Autodesk Inventor part; units mm, degrees
ref_plane "YZ Plane" through (0, 0, 0) normal (1, 0, 0) x (0, 1, 0)
ref_plane "XZ Plane" through (0, 0, 0) normal (0, 1, 0) x (-1, 0, 0)
ref_plane "XY Plane" through (0, 0, 0) normal (0, 0, 1) x (1, 0, 0)
sketch "Skizze1" plane through (0, 0, 0) normal (0, 0, 1) x (1, 0, 0)
  line L0 (0, 0) -> (242, 0)
  line L1 (242, 0) -> (242, 85)
  line L2 (242, 85) -> (0, 85)
  line L3 (0, 85) -> (0, 0)
  line L4 (242, 42.5) -> (842, 42.5)
  line L5 (0, 42.5) -> (-937, 42.5)
  arc A0 (240, 0) -> (240, 85) centre (-210.5625, 42.5) ccw
  arc A1 (2, 85) -> (2, 0) centre (452.5625, 42.5) ccw
  dimension "d0" = 85
  dimension "d1" = 242
  dimension "d2" = 2
  dimension "d3" = 2
  dimension "d4" = 2
  dimension "d7" = 452.5625
  dimension "d8" = 452.5625
extrude "Extrusion1" add sketch "Skizze1" against normal blind 2.5 contours A1 L2 A0 L0
sketch "Skizze2" plane through (0, 0, 0) normal (0, 0, 1) x (1, 0, 0)
  line L0 (2, 0) -> (240, 0)
  line L1 (240, 85) -> (2, 85)
  line L2 (121, 0) -> (121, 85)
  point P0 (0, 0)
  point P1 (3.1, 42.5)
  point P2 (238.9, 42.5)
  dimension "d11" = 42.5
  dimension "d12" = 42.5
  dimension "d13" = 235.8
  dimension "d14" = 117.9
  dimension "d15" = 117.9
hole "Bohrung1" at (3.1, 42.5, 0) at (238.9, 42.5, 0) direction (0, 0, -1) diameter 3.3 depth 8 tip angle 118
sketch "Skizze3" plane through (0, 0, 0) normal (0, 0, 1) x (1, 0, 0)
  line L0 (2, 0) -> (240, 0)
  line L1 (240, 85) -> (2, 85)
  arc A0 (2, 85) -> (2, 0) centre (452.5625, 42.5) ccw
  line L2 (8.1386, 91.5936) -> (-1.2688, 78.1585)
  line L3 (-1.2688, 78.1585) -> (-1.2688, 91.5936)
  line L4 (-1.2688, 91.5936) -> (8.1386, 91.5936)
  line L5 (-1.7926, 7.5896) -> (9.0296, -7.8661)
  line L6 (9.0296, -7.8661) -> (-1.7926, -7.8661)
  line L7 (-1.7926, -7.8661) -> (-1.7926, 7.5896)
  line L8 (121, 0) -> (121, 85)
  line L9 (233.8614, 91.5936) -> (243.2688, 78.1585)
  line L10 (243.2688, 78.1585) -> (243.2688, 91.5936)
  line L11 (243.2688, 91.5936) -> (233.8614, 91.5936)
  line L12 (243.7926, 7.5896) -> (232.9704, -7.8661)
  line L13 (232.9704, -7.8661) -> (243.7926, -7.8661)
  line L14 (243.7926, -7.8661) -> (243.7926, 7.5896)
  point P0 (0, 0)
  point P1 (1.7712, 82.5)
  point P2 (1.7712, 2.5)
  point P3 (242, 0)
  point P4 (240.2288, 82.5)
  point P5 (240.2288, 2.5)
  dimension "d23" = 55
  dimension "d24" = 55
  dimension "d25" = 2.5
  dimension "d26" = 2.5
extrude "Extrusion2" cut sketch "Skizze3" against normal blind 5 contours A0 L5 L0 | L0 L5 L6 L7 A0 | L9 L11 L10 | L12 L14 L13 | L2 L3 L4 L1 A0 | A0 L1 L2
sketch "Sketch7" plane through (0, 0, 0) normal (0, 0, 1) x (1, 0, 0)
  point P0 (0, 0)
sketch "Sketch9" plane through (0, 0, -2.5) normal (0, 0, -1) x (-1, 0, 0)
  line L0 (-238.4783, 85) -> (-3.5217, 85)
  line L1 (-214.9283, 63.0506) -> (-222.0283, 63.0506) construction
  line L2 (-222.0283, 63.0506) -> (-222.0283, 66.9494)
  line L3 (-222.0283, 66.9494) -> (-214.9283, 66.9494) construction
  line L4 (-214.9283, 66.9494) -> (-214.9283, 63.0506)
  line L5 (-214.9283, 63.0506) -> (-222.0283, 66.9494) construction
  line L6 (-222.0283, 63.0506) -> (-214.9283, 66.9494) construction
  arc A0 (-222.0283, 63.0506) -> (-214.9283, 63.0506) centre (-218.4783, 65) ccw
  arc A1 (-214.9283, 66.9494) -> (-222.0283, 66.9494) centre (-218.4783, 65) ccw
  line L7 (-194.9283, 63.0506) -> (-202.0283, 63.0506) construction
  line L8 (-202.0283, 63.0506) -> (-202.0283, 66.9494)
  line L9 (-202.0283, 66.9494) -> (-194.9283, 66.9494) construction
  line L10 (-194.9283, 66.9494) -> (-194.9283, 63.0506)
  line L11 (-194.9283, 63.0506) -> (-202.0283, 66.9494) construction
  line L12 (-202.0283, 63.0506) -> (-194.9283, 66.9494) construction
  arc A2 (-202.0283, 63.0506) -> (-194.9283, 63.0506) centre (-198.4783, 65) ccw
  arc A3 (-194.9283, 66.9494) -> (-202.0283, 66.9494) centre (-198.4783, 65) ccw
  line L13 (-174.9283, 63.0506) -> (-182.0283, 63.0506) construction
  line L14 (-182.0283, 63.0506) -> (-182.0283, 66.9494)
  line L15 (-182.0283, 66.9494) -> (-174.9283, 66.9494) construction
  line L16 (-174.9283, 66.9494) -> (-174.9283, 63.0506)
  line L17 (-174.9283, 63.0506) -> (-182.0283, 66.9494) construction
  line L18 (-182.0283, 63.0506) -> (-174.9283, 66.9494) construction
  arc A4 (-182.0283, 63.0506) -> (-174.9283, 63.0506) centre (-178.4783, 65) ccw
  arc A5 (-174.9283, 66.9494) -> (-182.0283, 66.9494) centre (-178.4783, 65) ccw
  line L19 (-154.9283, 63.0506) -> (-162.0283, 63.0506) construction
  line L20 (-162.0283, 63.0506) -> (-162.0283, 66.9494)
  line L21 (-162.0283, 66.9494) -> (-154.9283, 66.9494) construction
  line L22 (-154.9283, 66.9494) -> (-154.9283, 63.0506)
  line L23 (-154.9283, 63.0506) -> (-162.0283, 66.9494) construction
  line L24 (-162.0283, 63.0506) -> (-154.9283, 66.9494) construction
  arc A6 (-162.0283, 63.0506) -> (-154.9283, 63.0506) centre (-158.4783, 65) ccw
  arc A7 (-154.9283, 66.9494) -> (-162.0283, 66.9494) centre (-158.4783, 65) ccw
  line L25 (-134.9283, 63.0506) -> (-142.0283, 63.0506) construction
  line L26 (-142.0283, 63.0506) -> (-142.0283, 66.9494)
  line L27 (-142.0283, 66.9494) -> (-134.9283, 66.9494) construction
  line L28 (-134.9283, 66.9494) -> (-134.9283, 63.0506)
  line L29 (-134.9283, 63.0506) -> (-142.0283, 66.9494) construction
  line L30 (-142.0283, 63.0506) -> (-134.9283, 66.9494) construction
  arc A8 (-142.0283, 63.0506) -> (-134.9283, 63.0506) centre (-138.4783, 65) ccw
  arc A9 (-134.9283, 66.9494) -> (-142.0283, 66.9494) centre (-138.4783, 65) ccw
  line L31 (-114.9283, 63.0506) -> (-122.0283, 63.0506) construction
  line L32 (-122.0283, 63.0506) -> (-122.0283, 66.9494)
  line L33 (-122.0283, 66.9494) -> (-114.9283, 66.9494) construction
  line L34 (-114.9283, 66.9494) -> (-114.9283, 63.0506)
  line L35 (-114.9283, 63.0506) -> (-122.0283, 66.9494) construction
  line L36 (-122.0283, 63.0506) -> (-114.9283, 66.9494) construction
  arc A10 (-122.0283, 63.0506) -> (-114.9283, 63.0506) centre (-118.4783, 65) ccw
  arc A11 (-114.9283, 66.9494) -> (-122.0283, 66.9494) centre (-118.4783, 65) ccw
  circle A12 centre (-218.4783, 50) radius 2.4
  circle A13 centre (-198.4783, 50) radius 2.4
  circle A14 centre (-178.4783, 50) radius 2.4
  circle A15 centre (-158.4783, 50) radius 2.4
  circle A16 centre (-138.4783, 50) radius 2.4
  circle A17 centre (-118.4783, 50) radius 2.4
  point P0 (0, 0)
  dimension "d97" = 20
  dimension "d98" = 20
  dimension "d99" = 7.1
  dimension "d100" = 4.05
  dimension "d103" = 20
  dimension "d108" = 15
  dimension "d109" = 4.8
  dimension "d112" = 20
extrude "Extrusion6" cut sketch "Sketch9" against normal blind 3
properties part number "Frontplatte Apra Xdream 418"
Could you check a few things on this model? Use its own coordinates, in mm. Coordinates: 2 decimals unless noted, no trailing zeros. Write each loop counter-clockwise with the first axis right and the second up, starting at its lowest first coordinate (ties: lowest second). Pieces come first, ordered by that corner, then holes. Notation, with made-up numbers: M 72,-0.5 L 96,-0.5 A12 cw 96,21.5 Z; hole C -5.5,47 d5. An arc over 180 degrees is marked long. Answer as CSV lines item,"result". Start each with the question number.
1) For P1, Ø4, axis at x = 118.48, y = 50, coming from the +Z side; P2, Ø1.5, axis at y = 24.5, z = -2, coming from the -X side; P3, Ø1, axis at y = 10, z = -1, coming from the -X side, each with a flat end and sliding along its axis, tell me the tip position at first contact or that it passes through.
2) I want a section at A-A, the plane y = 50. Please give me the cut outline in (x, z), and give its area (3 significant figures).
3) Please list where these lines run through material, in increasing order: line 1 (Y direction, x = 160, z = -1.55); line 2 (X direction, y = 12, z = -0.15); line 3 (X direction, y = 55, z = -2). Write a range as from..to.
4) I want a section at C-C, the plane z = -1. Give the number of separate pieces and of enclosed holes in the cut face, and give its area (3 significant figures).
5) I want a section at B-B, the plane x = 218.5. Please give me the cut outline in (y, z), and give its area (3 significant figures).
6) We'd pull the mould along Y, two halves only. Please class faces 1 (the cylindrical face through (120.383, 48.54, -1.268)), 2 (the cylindrical face through (140.383, 48.54, -1.268)), 3 (the flat face through (119, 43, -2.5)): +Y half, -Y half, draft (parallel to the pull), parting line (faces both ways), or undercut.
Data:
1,P1,"passes through"
1,P2,"stops at x = 0.33"
1,P3,"stops at x = 1.13"
2,outline,"M 0.06,-2.5 L 116.08,-2.5 L 116.08,0 L 0.06,0 Z; M 120.88,-2.5 L 136.08,-2.5 L 136.08,0 L 120.88,0 Z; M 140.88,-2.5 L 156.08,-2.5 L 156.08,0 L 140.88,0 Z; M 160.88,-2.5 L 176.08,-2.5 L 176.08,0 L 160.88,0 Z; M 180.88,-2.5 L 196.08,-2.5 L 196.08,0 L 180.88,0 Z; M 200.88,-2.5 L 216.08,-2.5 L 216.08,0 L 200.88,0 Z; M 220.88,-2.5 L 241.94,-2.5 L 241.94,0 L 220.88,0 Z"
2,area,"533 mm^2"
3,line 1,"y = 0..48.14, 51.86..61.25, 68.75..85"
3,line 2,"x = 1.03..240.97"
3,line 3,"x = 0.17..241.83"
4,separate pieces,"1"
4,enclosed holes,"14"
4,area,"20,000 mm^2"
5,outline,"M 0,-2.5 L 47.6,-2.5 L 47.6,0 L 0,0 Z; M 52.4,-2.5 L 60.95,-2.5 L 60.95,0 L 52.4,0 Z; M 69.05,-2.5 L 85,-2.5 L 85,0 L 69.05,0 Z"
5,area,"180 mm^2"
6,face 1,"undercut"
6,face 2,"undercut"
6,face 3,"draft"
